Verification items for the finished model (mm, model axes). Face numbers are marked on the shaded views. A direction names the side the tool comes from. Coordinates: 2 decimals unless noted, no trailing zeros. Order: outer loops, then holes, each group sorted by start corner. A loop starts at its lowest first (then second) coordinate and runs counter-clockwise, first axis right, second up. Notation, with made-up numbers: M 35.5,53 L 40.5,53 A33 ccw 40.5,81 Z; hole C -8,-8.5 d10. An arc over 180 degrees is marked long. Return JSON: item names as keys, results as strings. Group by question number.
1. Set-up check for the marked faces 1, 2 and 3: record each of +Z, -Z, +X, -X, +Y, -Y from which the full face is reachable in a straight line by a thin tool's end or side.
2. Mould release check, pull along X, two halves, no side actions. Record for the marked faces 4, 5 and 6: +X half, -X half, draft (parallel to the pull), parting line (faces both ways), or undercut.
3. Section check A-A, the plane z = 7. Record the cut outline in (x, y).
4. Gauge pin test, flat ends, axial feed: pin 1 (3 mm diameter, centred on x = 7, z = 6, fed in from +Y); pin 2 (1.5 mm diameter, centred on x = 11, y = 24.5, fed in from -Z); pin 3 (1 mm diameter, centred on x = 21, z = 10, fed in from +Y); pin 4 (6 mm diameter, centred on y = 14, z = 11, fed in from -X). Record the tip position at first contact, or that the pin passes through.
5. Section check C-C, the plane y = 20. Record the cut outline in (x, z).
6. Material ranges on line 1 along Z through (x, y) = (37.25, 1.65); line 2 along X through (y, z) = (8.5, 4.25); line 3 along Z through (x, y) = (5, 3), recorded low to high.
7. Section check D-D, the plane z = 12. Record the cut outline in (x, y), plus the area to 3 significant figures.
8. Section check B-B, the plane x = 5.5. Record the cut outline in (y, z).
```python
from build123d import *

# Parameters (mm, degrees)
BOSS_EXTRUDE1_DEPTH = 14
SKETCH2_R           = 4
CUT_EXTRUDE1_DEPTH  = 56.303706928
SKETCH3_R           = 2.5
CUT_EXTRUDE2_DEPTH  = 14
SKETCH4_R           = 2.5
CUT_EXTRUDE3_DEPTH  = 14
SKETCH5_W           = 2
SKETCH5_H           = 14
CUT_EXTRUDE4_DEPTH  = 3


with BuildPart() as part:
    # Sketch1 → Boss-Extrude1 (new body)
    with BuildSketch(Plane.XY):
        Polygon((0, 0), (42.5, 0), (42.5, 5), (32.5, 5), (32.5, 32.5), (10, 32.5), (10, 5), (0, 5), align=None)
    extrude(amount=BOSS_EXTRUDE1_DEPTH)

    # Sketch2 → Cut-Extrude1 (cut, through all)
    with BuildSketch(Plane.XY.offset(14)):
        with Locations((21.25, 20)):
            Circle(SKETCH2_R)
    extrude(amount=-CUT_EXTRUDE1_DEPTH, mode=Mode.SUBTRACT)

    # Sketch3 → Cut-Extrude2 (cut)
    with BuildSketch(Plane(origin=(0, 5, 0), x_dir=(1, 0, 0), z_dir=(0, 1, 0))):
        with Locations(Location((5.5, -7, 0), (0, 0, 270))):
            Circle(SKETCH3_R)
    extrude(amount=-CUT_EXTRUDE2_DEPTH, mode=Mode.SUBTRACT)

    # Sketch4 → Cut-Extrude3 (cut)
    with BuildSketch(Plane(origin=(0, 5, 0), x_dir=(1, 0, 0), z_dir=(0, 1, 0))):
        with Locations(Location((37.25, -7, 0), (0, 0, 180))):
            Circle(SKETCH4_R)
    extrude(amount=-CUT_EXTRUDE3_DEPTH, mode=Mode.SUBTRACT)

    # Sketch5 → Cut-Extrude4 (cut)
    with BuildSketch(Plane(origin=(0, 32.5, 0), x_dir=(1, 0, 0), z_dir=(0, 1, 0))):
        with Locations((21.25, -7)):
            Rectangle(SKETCH5_W, SKETCH5_H)
    extrude(amount=-CUT_EXTRUDE4_DEPTH, mode=Mode.SUBTRACT)


solid = part.part
```
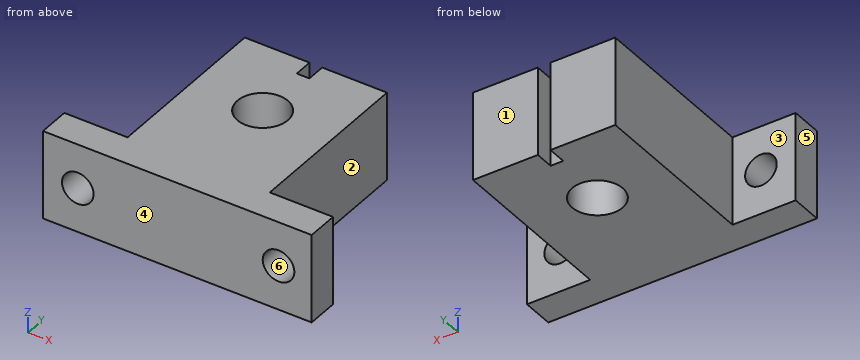
Answers follow:
{
 "1": {"face 1": "+Z, -Z, +X, -X, +Y", "face 2": "+Z, -Z, +X, +Y", "face 3": "+Z, -Z, -X, +Y"},
 "2": {"face 4": "draft", "face 5": "-X half", "face 6": "undercut"},
 "3": {"outline": "M 0,0 L 3,0 L 3,5 L 0,5 Z; M 8,0 L 34.75,0 L 34.75,5 L 32.5,5 L 32.5,32.5 L 22.25,32.5 L 22.25,29.5 L 20.25,29.5 L 20.25,32.5 L 10,32.5 L 10,5 L 8,5 Z; M 39.75,0 L 42.5,0 L 42.5,5 L 39.75,5 Z; hole C 21.25,20 d8"},
 "4": {"pin 1": "y = 5", "pin 2": "z = 0", "pin 3": "y = 29.5", "pin 4": "x = 10"},
 "5": {"outline": "M 10,0 L 17.25,0 L 17.25,14 L 10,14 Z; M 25.25,0 L 32.5,0 L 32.5,14 L 25.25,14 Z"},
 "6": {"line 1": "0 to 4.5, 9.5 to 14", "line 2": "10 to 32.5", "line 3": "0 to 4.55, 9.45 to 14"},
 "7": {"outline": "M 0,0 L 42.5,0 L 42.5,5 L 32.5,5 L 32.5,32.5 L 22.25,32.5 L 22.25,29.5 L 20.25,29.5 L 20.25,32.5 L 10,32.5 L 10,5 L 0,5 Z; hole C 21.25,20 d8", "area": "775 mm^2"},
 "8": {"outline": "M 0,0 L 5,0 L 5,4.5 L 0,4.5 Z; M 0,9.5 L 5,9.5 L 5,14 L 0,14 Z"}
}
